Source: CAD feature listing. Evaluate the final solid. Frame: model axes, mm. Face numbers are marked on the shaded views. Round coordinates to 2 decimals unless told otherwise and drop trailing zeros. Write each loop counter-clockwise with the first axis right and the second up, starting at its lowest first coordinate (ties: lowest second). Pieces come first, ordered by that corner, then holes. Notation, with made-up numbers: (-34.75, 39.25) -> (-30.75, 39.25) arc R27 cw to (-30.75, 67.25) -> close; hole circle Ø5 at (68.25, 34). An arc over 180 degrees is marked (long way). Return JSON: item names as keys, results as strings. Group by question number.
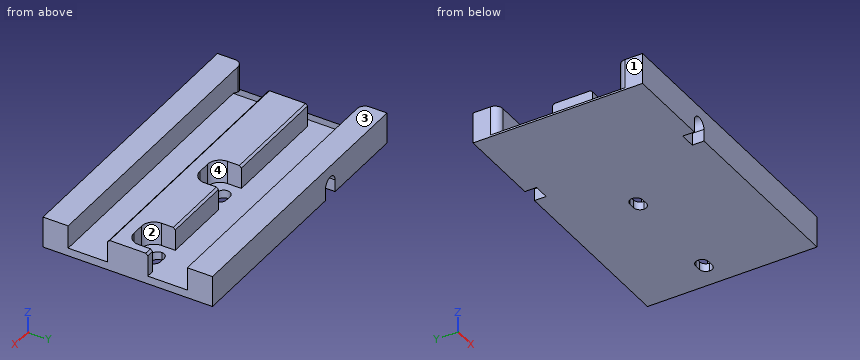
from build123d import *

# Parameters (mm, degrees)
F0_W      = 185.72
F0_H      = 110.42
F1_DEPTH  = 5.2
F3_DEPTH  = 110.42
F4_W      = 185.72
F4_H      = 16.4
F5_DEPTH  = 20.3
F6_W      = 24.4
F6_H      = 17
F6_W_2    = 24.3
F7_DEPTH  = 15.1
F8_R      = 8
F9_R      = 8
F10_R     = 5
F11_SIZE  = 1.3
F14_DEPTH = 7.6
F16_DEPTH = 7.6
F17_DEPTH = 20.301


with BuildPart() as f1:
    # F0 (on Top) → F1 (new body)
    with BuildSketch(Plane.XY):
        with Locations((-8.2149282098, -9.908063139)):
            Rectangle(F0_W, F0_H)
    extrude(amount=F1_DEPTH)

    # F2 (on face) → F3 (cut, through all)
    with BuildSketch(Plane.XZ.offset(65.118063139)):
        Polygon((-91.0749282098, 5.2), (-101.0749282098, 5.2), (-101.0749282098, 1.2), align=None)
    extrude(amount=-F3_DEPTH, mode=Mode.SUBTRACT)

    # F4 (on face) → F5 (join)
    with BuildSketch(Plane(origin=(0, 0, 0), x_dir=(1, 0, 0), z_dir=(0, 0, -1))):
        with Locations((-8.2149282098, 56.918063139)):
            Rectangle(F4_W, F4_H)
        with Locations((-8.2149282098, -37.101936861)):
            Rectangle(F4_W, F4_H)
        Polygon((84.6450717902, 9.908063139), (84.6450717902, 22.958063139), (-85.3549282098, 22.958063139), (-85.3549282098, 9.908063139), (-85.3549282098, -3.141936861), (84.6450717902, -3.141936861), align=None)
    extrude(amount=-F5_DEPTH)

    # F6 (on face) → F7 (cut)
    with BuildSketch(Plane.XY.offset(20.3)):
        with Locations((-2.7149282098, -5.358063139)):
            Rectangle(F6_W, F6_H)
        with Locations((67.4950717902, -5.358063139)):
            Rectangle(F6_W_2, F6_H)
    extrude(amount=-F7_DEPTH, mode=Mode.SUBTRACT)

    # F8
    f8_edges = [f1.edges().sort_by_distance(p)[0] for p in [
        (-14.914928, -13.858063, 12.75),
    ]]
    fillet(f8_edges, radius=F8_R)

    # F9
    f9_edges = [f1.edges().sort_by_distance(p)[0] for p in [
        (9.485072, -13.858063, 12.75),
        (79.645072, -13.858063, 12.75),
        (55.345072, -13.858063, 12.75),
    ]]
    fillet(f9_edges, radius=F9_R)

    # F10
    f10_edges = [f1.edges().sort_by_distance(p)[0] for p in [
        (-101.074928, 28.901937, 10.75),
        (-101.074928, -48.718063, 10.75),
    ]]
    fillet(f10_edges, radius=F10_R)

    # F11
    f11_edges = [f1.edges().sort_by_distance(p)[0] for p in [
        (-50.134928, 3.141937, 20.3),
        (32.415072, 3.141937, 20.3),
        (82.145072, 3.141937, 20.3),
        (-0.354928, -22.958063, 20.3),
    ]]
    chamfer(f11_edges, length=F11_SIZE)

    # F13 (on face) → F14 (cut)
    with BuildSketch(Plane.XZ.offset(65.118063139)):
        with BuildLine():
            Line((-45.8749282098, 7.9100113362), (-45.8749282098, 0))
            Line((-45.8749282098, 0), (-40.7749282098, 0))
            Line((-40.7749282098, 0), (-40.7749282098, 2.8100113362))
            ThreePointArc((-40.7749282098, 2.8100113362), (-44.3811727938, 4.3037667522), (-45.8749282098, 7.9100113362))
        make_face()
        with BuildLine():
            Line((-40.7749282098, 2.8100113362), (-40.7749282098, 0))
            Line((-40.7749282098, 0), (-35.6749282098, 0))
            Line((-35.6749282098, 0), (-35.6749282098, 7.9100113362))
            ThreePointArc((-35.6749282098, 7.9100113362), (-37.1686836257, 4.3037667522), (-40.7749282098, 2.8100113362))
        make_face()
        with BuildLine():
            Line((-40.7749282098, 7.9100113362), (-45.8749282098, 7.9100113362))
            ThreePointArc((-45.8749282098, 7.9100113362), (-44.3811727938, 4.3037667522), (-40.7749282098, 2.8100113362))
            Line((-40.7749282098, 2.8100113362), (-40.7749282098, 7.9100113362))
        make_face()
        with BuildLine():
            ThreePointArc((-35.6749282098, 7.9100113362), (-40.7749282098, 13.0100113362), (-45.8749282098, 7.9100113362))
            Line((-45.8749282098, 7.9100113362), (-40.7749282098, 7.9100113362))
            Line((-40.7749282098, 7.9100113362), (-35.6749282098, 7.9100113362))
        make_face()
        with BuildLine():
            Line((-40.7749282098, 7.9100113362), (-40.7749282098, 2.8100113362))
            ThreePointArc((-40.7749282098, 2.8100113362), (-37.1686836257, 4.3037667522), (-35.6749282098, 7.9100113362))
            Line((-35.6749282098, 7.9100113362), (-40.7749282098, 7.9100113362))
        make_face()
    extrude(amount=-F14_DEPTH, mode=Mode.SUBTRACT)

    # F15 (on face) → F16 (cut)
    with BuildSketch(Plane(origin=(0, 45.301936861, 0), x_dir=(-1, 0, 0), z_dir=(0, 1, 0))):
        with BuildLine():
            Line((40.7749282098, 0), (45.8749282098, 0))
            Line((45.8749282098, 0), (45.8749282098, 7.9))
            ThreePointArc((45.8749282098, 7.9), (44.3811727938, 4.2937554159), (40.7749282098, 2.8))
            Line((40.7749282098, 2.8), (40.7749282098, 0))
        make_face()
        with BuildLine():
            Line((35.6749282098, 0), (40.7749282098, 0))
            Line((40.7749282098, 0), (40.7749282098, 2.8))
            ThreePointArc((40.7749282098, 2.8), (37.1686836257, 4.2937554159), (35.6749282098, 7.9))
            Line((35.6749282098, 7.9), (35.6749282098, 0))
        make_face()
        with BuildLine():
            ThreePointArc((40.7749282098, 2.8), (44.3811727938, 4.2937554159), (45.8749282098, 7.9))
            Line((45.8749282098, 7.9), (40.7749282098, 7.9))
            Line((40.7749282098, 7.9), (40.7749282098, 2.8))
        make_face()
        with BuildLine():
            ThreePointArc((35.6749282098, 7.9), (37.1686836257, 4.2937554159), (40.7749282098, 2.8))
            Line((40.7749282098, 2.8), (40.7749282098, 7.9))
            Line((40.7749282098, 7.9), (35.6749282098, 7.9))
        make_face()
        with BuildLine():
            Line((40.7749282098, 7.9), (45.8749282098, 7.9))
            ThreePointArc((45.8749282098, 7.9), (40.7749282098, 13), (35.6749282098, 7.9))
            Line((35.6749282098, 7.9), (40.7749282098, 7.9))
        make_face()
    extrude(amount=-F16_DEPTH, mode=Mode.SUBTRACT)

    # F12 (on face) → F17 (cut, through all)
    with BuildSketch(Plane(origin=(0, 0, 0), x_dir=(1, 0, 0), z_dir=(0, 0, -1))):
        with BuildLine():
            ThreePointArc((-0.9549282098, -1.951936861), (1.9795649321, -0.7364300029), (3.1950717902, 2.198063139))
            Line((3.1950717902, 2.198063139), (-0.7049282098, 2.198063139))
            ThreePointArc((-0.7049282098, 2.198063139), (-1.2971901643, 0.0614770771), (-2.9049282098, -1.4652686778))
            ThreePointArc((-2.9049282098, -1.4652686778), (-1.9598344144, -1.8284320516), (-0.9549282098, -1.951936861))
        make_face()
        with BuildLine():
            Line((-0.7049282098, 2.198063139), (3.1950717902, 2.198063139))
            ThreePointArc((3.1950717902, 2.198063139), (1.9795649321, 5.132556281), (-0.9549282098, 6.348063139))
            ThreePointArc((-0.9549282098, 6.348063139), (-1.9598344144, 6.2245583296), (-2.9049282098, 5.8613949558))
            ThreePointArc((-2.9049282098, 5.8613949558), (-1.2971901643, 4.334649201), (-0.7049282098, 2.198063139))
        make_face()
        with BuildLine():
            ThreePointArc((69.0750717902, -1.951936861), (72.0095649321, -0.7364300029), (73.2250717902, 2.198063139))
            Line((73.2250717902, 2.198063139), (69.3250717902, 2.198063139))
            ThreePointArc((69.3250717902, 2.198063139), (68.7328098357, 0.0614770771), (67.1250717902, -1.4652686778))
            ThreePointArc((67.1250717902, -1.4652686778), (68.0701655856, -1.8284320516), (69.0750717902, -1.951936861))
        make_face()
        with BuildLine():
            Line((69.3250717902, 2.198063139), (73.2250717902, 2.198063139))
            ThreePointArc((73.2250717902, 2.198063139), (72.0095649321, 5.132556281), (69.0750717902, 6.348063139))
            ThreePointArc((69.0750717902, 6.348063139), (68.0701655856, 6.2245583296), (67.1250717902, 5.8613949558))
            ThreePointArc((67.1250717902, 5.8613949558), (68.7328098357, 4.334649201), (69.3250717902, 2.198063139))
        make_face()
        with BuildLine():
            ThreePointArc((67.1250717902, -1.4652686778), (68.7328098357, 0.0614770771), (69.3250717902, 2.198063139))
            Line((69.3250717902, 2.198063139), (69.0750717902, 2.198063139))
            Line((69.0750717902, 2.198063139), (65.1750717902, 2.198063139))
            Line((65.1750717902, 2.198063139), (64.9250717902, 2.198063139))
            ThreePointArc((64.9250717902, 2.198063139), (65.5173337448, 0.0614770771), (67.1250717902, -1.4652686778))
        make_face()
        with BuildLine():
            Line((69.0750717902, 2.198063139), (69.3250717902, 2.198063139))
            ThreePointArc((69.3250717902, 2.198063139), (68.7328098357, 4.334649201), (67.1250717902, 5.8613949558))
            ThreePointArc((67.1250717902, 5.8613949558), (65.5173337448, 4.334649201), (64.9250717902, 2.198063139))
            Line((64.9250717902, 2.198063139), (65.1750717902, 2.198063139))
            Line((65.1750717902, 2.198063139), (69.0750717902, 2.198063139))
        make_face()
        with BuildLine():
            ThreePointArc((67.1250717902, 5.8613949558), (68.0701655856, 6.2245583296), (69.0750717902, 6.348063139))
            Line((69.0750717902, 6.348063139), (65.1750717902, 6.348063139))
            ThreePointArc((65.1750717902, 6.348063139), (66.1799779949, 6.2245583296), (67.1250717902, 5.8613949558))
        make_face()
        with BuildLine():
            Line((65.1750717902, -1.951936861), (69.0750717902, -1.951936861))
            ThreePointArc((69.0750717902, -1.951936861), (68.0701655856, -1.8284320516), (67.1250717902, -1.4652686778))
            ThreePointArc((67.1250717902, -1.4652686778), (66.1799779949, -1.8284320516), (65.1750717902, -1.951936861))
        make_face()
        with BuildLine():
            ThreePointArc((64.9250717902, 2.198063139), (65.5173337448, 4.334649201), (67.1250717902, 5.8613949558))
            ThreePointArc((67.1250717902, 5.8613949558), (66.1799779949, 6.2245583296), (65.1750717902, 6.348063139))
            ThreePointArc((65.1750717902, 6.348063139), (62.2405786483, 5.132556281), (61.0250717902, 2.198063139))
            Line((61.0250717902, 2.198063139), (64.9250717902, 2.198063139))
        make_face()
        with BuildLine():
            ThreePointArc((65.1750717902, -1.951936861), (66.1799779949, -1.8284320516), (67.1250717902, -1.4652686778))
            ThreePointArc((67.1250717902, -1.4652686778), (65.5173337448, 0.0614770771), (64.9250717902, 2.198063139))
            Line((64.9250717902, 2.198063139), (61.0250717902, 2.198063139))
            ThreePointArc((61.0250717902, 2.198063139), (62.2405786483, -0.7364300029), (65.1750717902, -1.951936861))
        make_face()
        with BuildLine():
            ThreePointArc((-2.9049282098, -1.4652686778), (-1.2971901643, 0.0614770771), (-0.7049282098, 2.198063139))
            ThreePointArc((-0.7049282098, 2.198063139), (-1.2971901643, 4.334649201), (-2.9049282098, 5.8613949558))
            ThreePointArc((-2.9049282098, 5.8613949558), (-5.1049282098, 2.198063139), (-2.9049282098, -1.4652686778))
        make_face()
        with BuildLine():
            ThreePointArc((-2.9049282098, 5.8613949558), (-1.9598344144, 6.2245583296), (-0.9549282098, 6.348063139))
            Line((-0.9549282098, 6.348063139), (-4.8549282098, 6.348063139))
            ThreePointArc((-4.8549282098, 6.348063139), (-3.8500220051, 6.2245583296), (-2.9049282098, 5.8613949558))
        make_face()
        with BuildLine():
            Line((-4.8549282098, -1.951936861), (-0.9549282098, -1.951936861))
            ThreePointArc((-0.9549282098, -1.951936861), (-1.9598344144, -1.8284320516), (-2.9049282098, -1.4652686778))
            ThreePointArc((-2.9049282098, -1.4652686778), (-3.8500220051, -1.8284320516), (-4.8549282098, -1.951936861))
        make_face()
        with BuildLine():
            ThreePointArc((-2.9049282098, -1.4652686778), (-5.1049282098, 2.198063139), (-2.9049282098, 5.8613949558))
            ThreePointArc((-2.9049282098, 5.8613949558), (-3.8500220051, 6.2245583296), (-4.8549282098, 6.348063139))
            ThreePointArc((-4.8549282098, 6.348063139), (-9.0049282098, 2.198063139), (-4.8549282098, -1.951936861))
            ThreePointArc((-4.8549282098, -1.951936861), (-3.8500220051, -1.8284320516), (-2.9049282098, -1.4652686778))
        make_face()
    extrude(amount=-F17_DEPTH, mode=Mode.SUBTRACT)


solid = f1.part
Item 1: Cut plane B-B on x = 42. Output: boundary loops of the cut face in (y, z), and give its area (3 significant figures).
Item 2: First-contact query: pin 1 Ø4.5 at (y, z) = (0, 14.5) entering from -X; pin 2 Ø1 at (y, z) = (-50.5, 14.5) entering from -X; pin 3 Ø3 at (x, z) = (-42, 5.5) entering from -Y. Flat tips, straight axial feed; report the tip coordinate or a pass-through.
Item 3: Pull-direction query (X, two-part tool) for the marked faces 1, 2, 3 and 4; classes: +X half, -X half, draft (parallel to the pull), parting line (faces both ways), or undercut.
Item 4: Material intervals for probe 1 along X at (y, z) = (-1.5, 13.5); probe 2 along Y at (x, z) = (-52, 5.25); probe 3 along X at (y, z) = (-9, 15.75), sorted ascending.
Item 5: Cut plane A-A on z = 11. Give the number of separate pieces and of enclosed holes in the cut face, and give its area (3 significant figures).
Item 6: Cut plane C-C on y = 19.5. Output: boundary loops of the cut face in (x, z), and give its area (3 significant figures).
Here are the results:
{
 "1": {"outline": "(-65.12, 0) -> (45.3, 0) -> (45.3, 20.3) -> (28.9, 20.3) -> (28.9, 5.2) -> (3.14, 5.2) -> (3.14, 19) -> (1.84, 20.3) -> (-21.66, 20.3) -> (-22.96, 19) -> (-22.96, 5.2) -> (-48.72, 5.2) -> (-48.72, 20.3) -> (-65.12, 20.3) -> close", "area": "1,460 mm^2"},
 "2": {"pin 1": "stops at x = -85.35", "pin 2": "stops at x = -100.27", "pin 3": "stops at y = -57.52"},
 "3": {"face 1": "-X half", "face 2": "undercut", "face 3": "draft", "face 4": "undercut"},
 "4": {"probe 1": "x = -85.35 to -14.91, 9.49 to 55.35, 79.65 to 84.65", "probe 2": "y = -65.12 to -48.72, -22.96 to 3.14, 28.9 to 45.3", "probe 3": "x = -85.35 to -14.27, 8.84 to 55.99, 79 to 84.65"},
 "5": {"separate pieces": "3", "enclosed holes": "0", "area": "9,620 mm^2"},
 "6": {"outline": "(-101.07, 0) -> (84.65, 0) -> (84.65, 5.2) -> (-91.07, 5.2) -> (-101.07, 1.2) -> close", "area": "946 mm^2"}
}
